Geometry: see drawing. Coordinates: mm, zero at the bounding-box minimum. A direction names the side the tool comes from. Coordinates: 2 decimals unless noted, no trailing zeros. Loops run counter-clockwise (first coordinate to the right, second up) from the corner with the lowest first, then second, coordinate; pieces in that order, holes last.
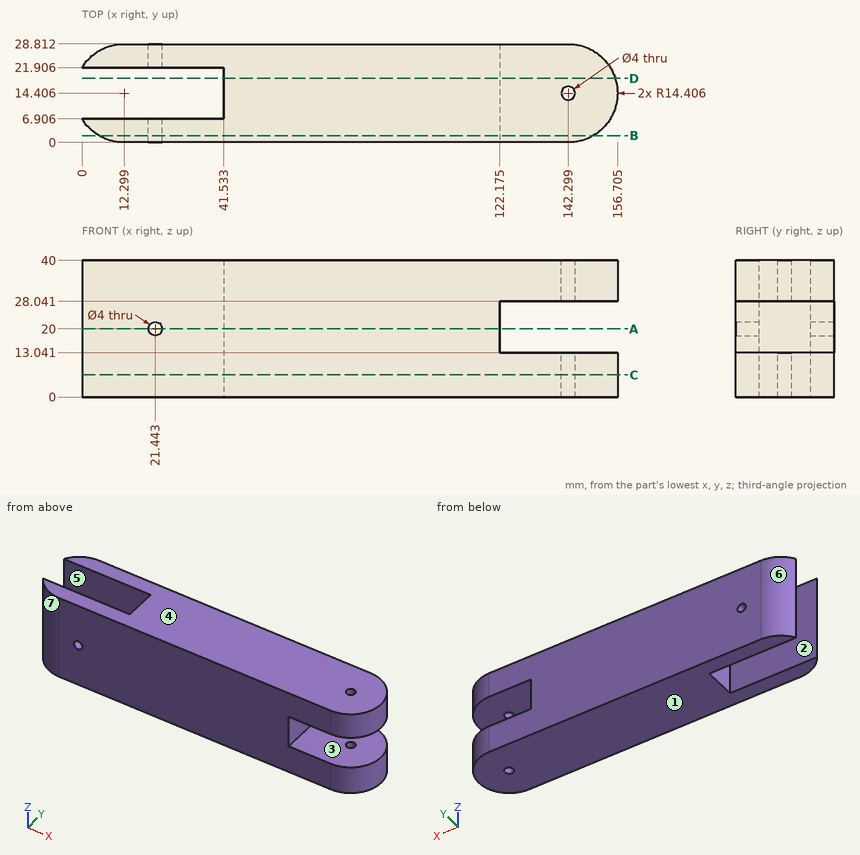
Item 1: Section query D-D (y = 18.75). Output: boundary loops of the cut face in (x, z) (1 decimal).
Result:
outline: (41.5, 0) - (156, 0) - (156, 13) - (122.2, 13) - (122.2, 28) - (156, 28) - (156, 40) - (41.5, 40) - close
Item 2: Section query A-A (z = 20). Output: boundary loops of the cut face in (x, y) (1 decimal), then the cut area to 3 significant figures.
Result:
outline: (0, 6.9) arc R14.4 ccw to (12.3, 0) - (19.4, 0) - (19.4, 6.9) - close; (0, 21.9) - (19.4, 21.9) - (19.4, 28.8) - (12.3, 28.8) arc R14.4 ccw to start; (23.4, 0) - (122.2, 0) - (122.2, 28.8) - (23.4, 28.8) - (23.4, 21.9) - (41.5, 21.9) - (41.5, 6.9) - (23.4, 6.9) - close
area: 2,790 mm2
Item 3: Line query: L1, parallel to Y at x = 14, z = 37 (1 decimal); L2, parallel to Z at x = 124.5, y = 17.25; L3, parallel to X at y = 27.5, z = 20 (1 decimal). Output: solid intervals per line, ascending.
Result:
L1: y = 0 to 6.9, 21.9 to 28.8
L2: z = 0 to 13.04, 28.04 to 40
L3: x = 6.3 to 19.4, 23.4 to 122.2
Item 4: Reachability of the marked faces 1, 2 and 3 from +Z, -Z, +X, -X, +Y, -Y: full face, straight path, thin tool, end or side. Return the list, or none.
Result:
face 1: -Z, +X, -X, +Y, -Y
face 2: +Z, -Z, -X
face 3: +X, +Y, -Y
Item 5: Section query C-C (z = 6.5). Output: boundary loops of the cut face in (x, y) (1 decimal), then the cut area to 3 significant figures.
Result:
outline: (0, 6.9) arc R14.4 ccw to (12.3, 0) - (142.3, 0) arc R14.4 ccw to (142.3, 28.8) - (12.3, 28.8) arc R14.4 ccw to (0, 21.9) - (41.5, 21.9) - (41.5, 6.9) - close; hole circle Ø4 at (142.3, 14.4)
area: 3,740 mm2
Item 6: Mould query, pull axis Y, two halves, no side actions, for the marked faces 4, 5, 6 and 7. Classes: +Y half, -Y half, draft (parallel to the pull), parting line (faces both ways), or undercut.
Result:
face 4: draft
face 5: undercut
face 6: +Y half
face 7: -Y half
Item 7: Contact query for flat-ended pins moving along their axis: P1, Ø2.5, axis at x = 142.3, y = 14.41, coming from the -Z side; P2, Ø4.5, axis at y = 13, z = 26, coming from the -X side; P3, Ø1, axis at y = 25.5, z = 36, coming from the -X side. Output: stop coordinate, or through.
Result:
P1: passes through
P2: stops at x = 41.53
P3: stops at x = 2.54
Item 8: Section query B-B (y = 2). Output: boundary loops of the cut face in (x, z) (1 decimal).
Result:
outline: (5, 0) - (149.6, 0) - (149.6, 13) - (122.2, 13) - (122.2, 28) - (149.6, 28) - (149.6, 40) - (5, 40) - close; hole circle Ø4 at (21.4, 20)
